Design review of the part shown in the three views and the two pictorial views. Dimensions are in mm from the part's minimum x, y and z. Coordinates: 2 decimals unless noted, no trailing zeros. Loops run counter-clockwise (first coordinate to the right, second up) from the corner with the lowest first, then second, coordinate; pieces in that order, holes last. Notation, with made-up numbers: M 85,86 L 134,86 A18 cw 134,112 Z; hole C -9.5,31.25 d8. An arc over 180 degrees is marked long. Use one line per item in the form item = value.
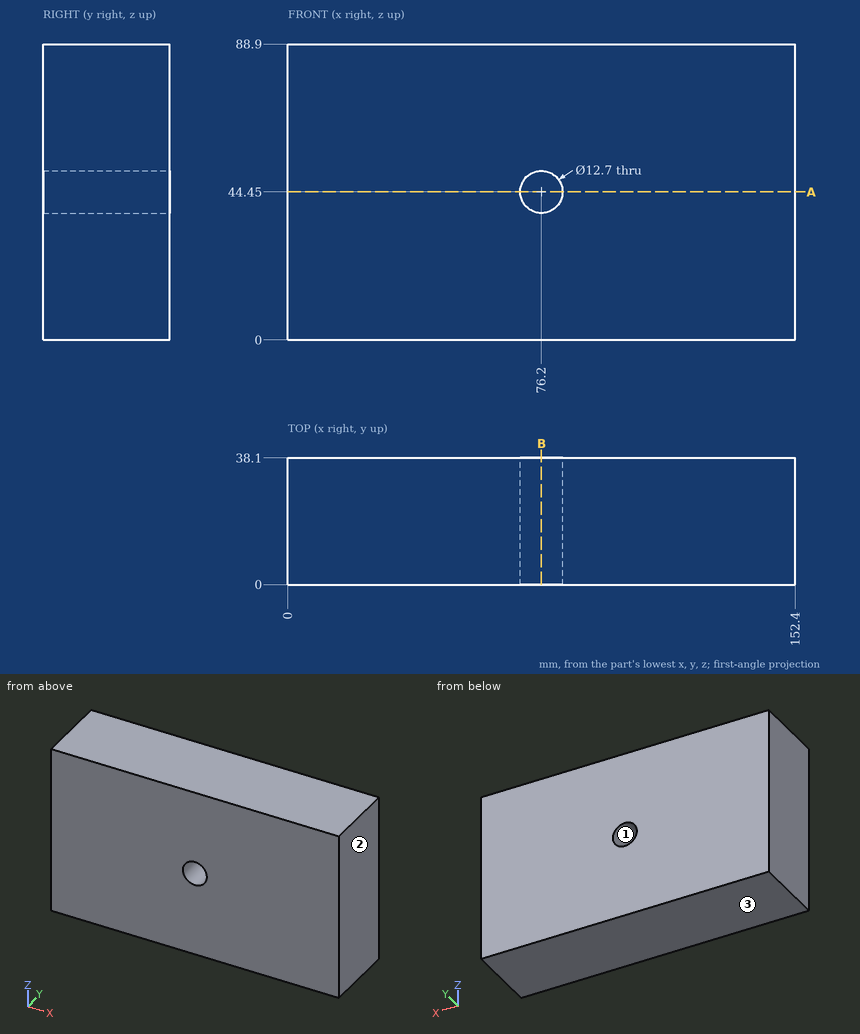
1. The part is to be moulded in two halves that separate along X. For the marked faces 1, 2 and 3, say which applies: pulls with the +X half, pulls with the -X half, needs draft (parallel to the pull), parting line crosses it, or undercut.
Response values:
face_1 = undercut
face_2 = pulls with the +X half
face_3 = needs draft
2. Insertion check: P1, Ø2, axis at y = 18, z = 25.5, coming from the -X side. The pin has a flat end and moves straight along its axis. Give the tip position at first contact, or say it passes through.
Response values:
P1 = 0
3. Wall thickness on line 1 along X through (y, z) = (15, 44); line 2 along Z through (x, y) = (76.2, 24); line 3 along X through (y, z) = (25, 39): over which ranges is each line inside the solid? List them lowest first. Write a range as from..to.
Response values:
line_1 = 0..69.87, 82.53..152.4
line_2 = 0..38.1, 50.8..88.9
line_3 = 0..72.94, 79.46..152.4
4. Add section B-B (x = 76.2). State the section outline as (y, z) points, then the cut area to 3 significant figures.
Response values:
outline = M 0,0 L 38.1,0 L 38.1,38.1 L 0,38.1 Z; M 0,50.8 L 38.1,50.8 L 38.1,88.9 L 0,88.9 Z
area = 2,900 mm^2
5. Add section A-A (z = 44.45). State the section outline as (x, y) points, then the cut area to 3 significant figures.
Response values:
outline = M 0,0 L 69.85,0 L 69.85,38.1 L 0,38.1 Z; M 82.55,0 L 152.4,0 L 152.4,38.1 L 82.55,38.1 Z
area = 5,320 mm^2
